```python
from build123d import *

# Parameters (mm, degrees)
ESQUISSE1_W             = 30
ESQUISSE1_H             = 5
BOSS_EXTRU_1_DEPTH      = 40
ESQUISSE2_R             = 8
ENL_V_MAT_EXTRU_1_DEPTH = 51.249378106


with BuildPart() as part:
    # Esquisse1 → Boss.-Extru.1 (new body)
    with BuildSketch(Plane.XY):
        with Locations((15, 2.5)):
            Rectangle(ESQUISSE1_W, ESQUISSE1_H)
    extrude(amount=BOSS_EXTRU_1_DEPTH)

    # Esquisse2 → Enlèv. mat.-Extru.1 (cut, through all)
    with BuildSketch(Plane.XZ):
        with Locations(Location((15, 27, 0), (0, 0, 270))):
            Circle(ESQUISSE2_R)
    extrude(amount=-ENL_V_MAT_EXTRU_1_DEPTH, mode=Mode.SUBTRACT)


solid = part.part
```
Check sheet for the modelled part. Datum: model origin and axes. Units: mm. Give positions to 0.01 mm unless a question says otherwise; leave off trailing zeros. Order: outer loops, then holes, each group sorted by start corner. A loop starts at its lowest first (then second) coordinate and runs counter-clockwise, first axis right, second up. Notation, with made-up numbers: M -23,-26 L -12,-26 A31 ccw -12,13 Z; hole C 55.5,86 d9. An arc over 180 degrees is marked long. Answer in a Markdown table with one row per item.
1) Thickness scan on L1, parallel to X at y = 1.55, z = 27; L2, parallel to X at y = 0.9, z = 28; L3, parallel to Z at x = 13.5, y = 4.45. Record the ranges inside material, lowest first. Write a range as [from, to].
Filled sheet:
| item | result |
|---|---|
| L1 | x = [0, 7], [23, 30] |
| L2 | x = [0, 7.06], [22.94, 30] |
| L3 | z = [0, 19.14], [34.86, 40] |
2) Release check for a two-part mould opening along X. For faces 1 (the flat face through (0, 2, 20)), 2 (the flat face through (15, 0, 15)), 3 (the cylindrical face through (10.132, 2.465, 33.349)) record: +X half, -X half, draft (parallel to the pull), parting line (faces both ways), or undercut.
Filled sheet:
| item | result |
|---|---|
| face 1 | -X half |
| face 2 | draft |
| face 3 | undercut |
3) Cross-section at B-B, the plane x = 7.5. Enter the section's corners in (y, z).
Filled sheet:
| item | result |
|---|---|
| outline | M 0,0 L 5,0 L 5,24.22 L 0,24.22 Z; M 0,29.78 L 5,29.78 L 5,40 L 0,40 Z |
4) Cross-section at A-A, the plane z = 27. Enter the section's corners in (x, y), plus the area to 3 significant figures.
Filled sheet:
| item | result |
|---|---|
| outline | M 0,0 L 7,0 L 7,5 L 0,5 Z; M 23,0 L 30,0 L 30,5 L 23,5 Z |
| area | 70.0 mm2 |
